```python
from build123d import *

# Parameters (mm, degrees)
BOSS_EXTRUDE1_DEPTH = 6.35


with BuildPart() as part:
    # Sketch1 → Boss-Extrude1 (new body)
    with BuildSketch(Plane.XY):
        with BuildLine():
            Line((0, 5.08), (0, 36.068))
            Line((0, 36.068), (36.068, 36.068))
            Line((36.068, 36.068), (36.068, 5.08))
            ThreePointArc((36.068, 5.08), (34.580102448, 1.487897552), (30.988, 0))
            Line((30.988, 0), (5.08, 0))
            ThreePointArc((5.08, 0), (1.487897552, 1.487897552), (0, 5.08))
        make_face()
        with BuildLine():
            Line((11.43, 6.35), (24.638, 6.35))
            ThreePointArc((24.638, 6.35), (28.230102448, 7.837897552), (29.718, 11.43))
            Line((29.718, 11.43), (29.718, 24.638))
            ThreePointArc((29.718, 24.638), (28.230102448, 28.230102448), (24.638, 29.718))
            Line((24.638, 29.718), (11.43, 29.718))
            ThreePointArc((11.43, 29.718), (7.837897552, 28.230102448), (6.35, 24.638))
            Line((6.35, 24.638), (6.35, 11.43))
            ThreePointArc((6.35, 11.43), (7.837897552, 7.837897552), (11.43, 6.35))
        make_face(mode=Mode.SUBTRACT)
    extrude(amount=BOSS_EXTRUDE1_DEPTH)


solid = part.part
```
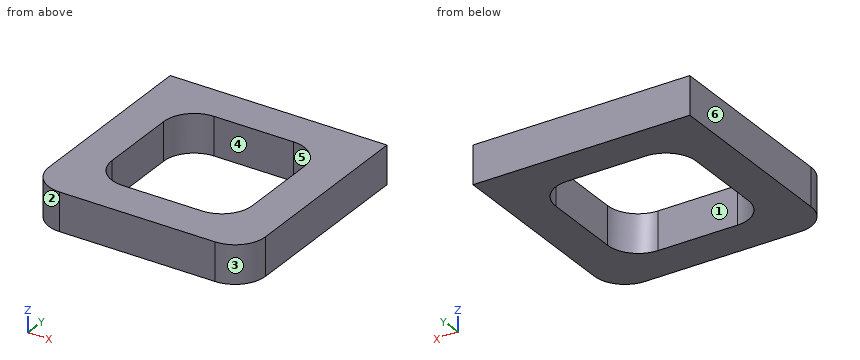
Can you work these out from the model? Positions are in its coordinate system, mm. Face numbers are marked on the shaded views. A direction names the side the tool comes from. Coordinates: 2 decimals unless noted, no trailing zeros. Order: outer loops, then holes, each group sorted by start corner. A loop starts at its lowest first (then second) coordinate and runs counter-clockwise, first axis right, second up.
1. If we section it at C-C (x = 8.5): Please give me the cut outline in (y, z), then the cut area to 3 significant figures.
2. If we section it at B-B (z = 5.5): Please give me the cut outline in (x, y).
3. For the marked faces 5 and 6, which set-ups out of +Z, -Z, +X, -X, +Y, -Y let a thin tool reach every point of the face, with its end or its side?
4. If we section it at A-A (y = 18): Please give me the cut outline in (x, z), then the cut area to 3 significant figures.
5. Thinking about a two-plate mould opening in X: for the marked faces 1, 2, 3 and 4, which applies, +X half, -X half, draft (parallel to the pull), parting line (faces both ways), or undercut?
6. I'm going to push a flat-ended pin straight in: pin 1 (3 mm diameter, centred on y = 17.5, z = 3.5, fed in from -X). Where does the tip first touch, or does it pass through?
7. I need wall thicknesses on line 1 (Y direction, x = 24, z = 0.5); line 2 (Y direction, x = 28, z = 0.75). Which ranges of each line are inside material? Lowest first, please.
Entries:
1. outline: (0, 0) - (7.28, 0) - (7.28, 6.35) - (0, 6.35) - close; (28.79, 0) - (36.07, 0) - (36.07, 6.35) - (28.79, 6.35) - close
1. area: 92.5 mm2
2. outline: (0, 5.08) arc R5.08 ccw to (5.08, 0) - (30.99, 0) arc R5.08 ccw to (36.07, 5.08) - (36.07, 36.07) - (0, 36.07) - close; hole (6.35, 11.43) arc R5.08 ccw to (11.43, 6.35) - (24.64, 6.35) arc R5.08 ccw to (29.72, 11.43) - (29.72, 24.64) arc R5.08 ccw to (24.64, 29.72) - (11.43, 29.72) arc R5.08 ccw to (6.35, 24.64) - close
3. face 5: +Z, -Z
3. face 6: +Z, -Z, -X, +Y, -Y
4. outline: (0, 0) - (6.35, 0) - (6.35, 6.35) - (0, 6.35) - close; (29.72, 0) - (36.07, 0) - (36.07, 6.35) - (29.72, 6.35) - close
4. area: 80.6 mm2
5. face 1: undercut
5. face 2: -X half
5. face 3: +X half
5. face 4: undercut
6. pin 1: stops at x = 0
7. line 1: y = 0 to 6.35, 29.72 to 36.07
7. line 2: y = 0 to 7.62, 28.45 to 36.07
